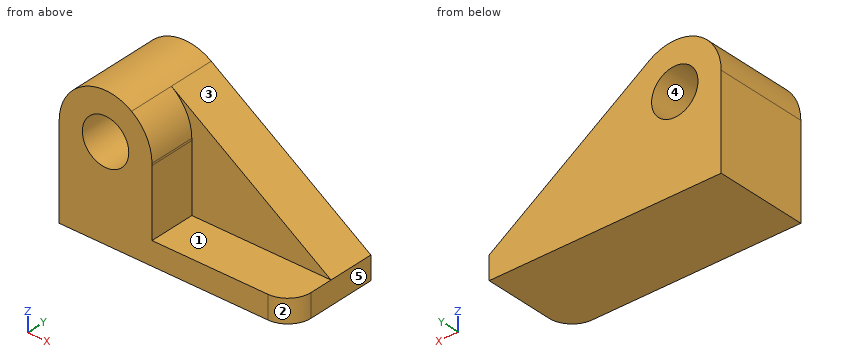
```python
from build123d import *

# Parameters (mm, degrees)
F0_R     = 12.7
F1_DEPTH = 25.4
F2_R     = 12.7
F3_DEPTH = 25.4
F4_R     = 12.7


with BuildPart() as f1:
    # F0 (on Front) → F1 (new body)
    with BuildSketch(Plane.XZ):
        with BuildLine():
            Line((61.366399, -2.3876), (-25.995728, 56.746728))
            ThreePointArc((-25.995728, 56.746728), (-52.13986, 58.148999), (-65.633601, 35.7124))
            Line((-65.633601, 35.7124), (-65.633601, -15.0876))
            Line((-65.633601, -15.0876), (61.366399, -15.0876))
            Line((61.366399, -15.0876), (61.366399, -2.3876))
        make_face()
        with Locations((-40.233601, 35.7124)):
            Circle(F0_R, mode=Mode.SUBTRACT)
    extrude(amount=F1_DEPTH)

    # F2 (on face) → F3 (join)
    with BuildSketch(Plane.XZ.offset(25.4)):
        with BuildLine():
            Line((-14.802516, -2.3876), (-14.858348, 34.591433))
            ThreePointArc((-14.858348, 34.591433), (-40.794221, 10.318588), (-65.633601, 35.7124))
            Line((-65.633601, 35.7124), (-65.633601, -2.3876))
            Line((-65.633601, -2.3876), (-65.633601, -15.0876))
            Line((-65.633601, -15.0876), (61.366399, -15.0876))
            Line((61.366399, -15.0876), (61.366399, -2.3876))
            Line((61.366399, -2.3876), (-14.802516, -2.3876))
        make_face()
        with BuildLine():
            ThreePointArc((-14.858348, 34.591433), (-14.839789, 35.15178), (-14.833601, 35.7124))
            ThreePointArc((-14.833601, 35.7124), (-17.797002, 47.618659), (-25.995728, 56.746728))
            ThreePointArc((-25.995728, 56.746728), (-52.13986, 58.148999), (-65.633601, 35.7124))
            ThreePointArc((-65.633601, 35.7124), (-40.794221, 10.318588), (-14.858348, 34.591433))
        make_face()
        with Locations((-40.233601, 35.7124)):
            Circle(F2_R, mode=Mode.SUBTRACT)
    extrude(amount=F3_DEPTH)

    # F4
    f4_edges = [f1.edges().sort_by_distance(p)[0] for p in [
        (61.366399, -50.8, -8.7376),
    ]]
    fillet(f4_edges, radius=F4_R)


solid = f1.part
```
The model under review builds one solid part; all positions refer to its coordinate system, in mm. Face numbers are marked on the shaded views. A direction names the side the tool comes from. Coordinates: 2 decimals unless noted, no trailing zeros. Write each loop counter-clockwise with the first axis right and the second up, starting at its lowest first coordinate (ties: lowest second). Pieces come first, ordered by that corner, then holes. Notation, with made-up numbers: (83, 68) -> (94, 68) arc R30 cw to (94, 96) -> close; hole circle Ø9 at (35.25, -33). An arc over 180 degrees is marked (long way). One line per item, written item: value. Start each with the question number.
Q1. Clearance check with flat-ended pins moving along their axes: P1, Ø8, axis at x = 38, y = -11, coming from the +Z side; P2, Ø4, axis at x = 15, z = 3.5, coming from the -Y side; P3, Ø4, axis at x = 3.5, y = -16.5, coming from the +Z side. State where each tip first meets the part, or that it passes through.
Q2. Add section A-A, the plane y = -31. Give the boundary of the cut face in (x, z), then the cut area to 3 significant figures.
Q3. For the marked faces 1 and 2, list the 3-axis set-ups (+Z, -Z, +X, -X, +Y, -Y) from which the entire face can be reached by the end or side of a thin tool; tool diameter is ignored.
Q4. Add section B-B, the plane z = 46. Give the boundary of the cut face in (x, y), then the cut area to 3 significant figures.
Q5. Add section D-D, the plane y = -42. Give the boundary of the cut face in (x, z), then the cut area to 3 significant figures.
Q6. The part is to be moulded in two halves that separate along Z. For the marked faces 3, 4 and 5, say which applies: +Z half, -Z half, draft (parallel to the pull), parting line (faces both ways), or undercut.
Q7. Add section C-C, the plane x = -3.5. Give the boundary of the cut face in (y, z), then the cut area to 3 significant figures.
Q8. To check wall thickness, follow probe 1 along Z at (x, y) = (-40, -20); probe 2 along X at (y, z) = (-5, 43); probe 3 along Z at (x, y) = (1.5, -39). State the ranges of each line that lie inside material, in increasing order.
Response:
1. P1: z = 16.14
1. P2: y = -25.4
1. P3: z = 38.14
2. outline: (-65.63, -15.09) -> (61.37, -15.09) -> (61.37, -2.39) -> (-14.8, -2.39) -> (-14.86, 34.59) arc R25.4 ccw to (-14.83, 35.71) arc R25.4 ccw to (-26, 56.75) arc R25.4 ccw to (-65.63, 35.71) -> close; hole circle Ø25.4 at (-40.23, 35.71)
2. area: 4,060 mm²
3. face 1: +Z, +X, -Y
3. face 2: +Z, -Z, +X, -Y
4. outline: (-63.46, -50.8) -> (-47.68, -50.8) -> (-47.68, 0) -> (-63.46, 0) -> close; (-32.79, -50.8) -> (-17.01, -50.8) -> (-17.01, -25.4) -> (-10.12, -25.4) -> (-10.12, 0) -> (-32.79, 0) -> close
4. area: 1,780 mm²
5. outline: (-65.63, -15.09) -> (60.75, -15.09) -> (60.75, -2.39) -> (-14.8, -2.39) -> (-14.86, 34.59) arc R25.4 ccw to (-14.83, 35.71) arc R25.4 ccw to (-26, 56.75) arc R25.4 ccw to (-65.63, 35.71) -> close; hole circle Ø25.4 at (-40.23, 35.71)
5. area: 4,050 mm²
6. face 3: +Z half
6. face 4: undercut
6. face 5: draft
7. outline: (-50.8, -15.09) -> (0, -15.09) -> (0, 41.52) -> (-25.4, 41.52) -> (-25.4, -2.39) -> (-50.8, -2.39) -> close
7. area: 1,760 mm²
8. probe 1: -15.09 to 23.01, 48.41 to 61.11
8. probe 2: -64.57 to -50.63, -29.83 to -5.69
8. probe 3: -15.09 to -2.39
